Source: CAD feature listing. Evaluate the final solid. Frame: model axes, mm. Face numbers are marked on the shaded views. A direction names the side the tool comes from. Give positions to 0.01 mm unless a question says otherwise; leave off trailing zeros. Order: outer loops, then holes, each group sorted by start corner. A loop starts at its lowest first (then second) coordinate and runs counter-clockwise, first axis right, second up. Notation, with made-up numbers: (37.25, 13) - (78.25, 13) arc R23 ccw to (78.25, 42) - close; hole circle Ø7 at (63, -11.75). An arc over 180 degrees is marked (long way). Answer as CSV lines item,"result".
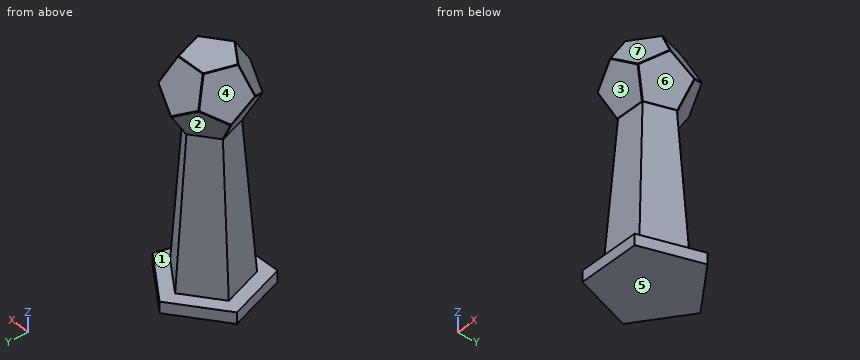
```python
from build123d import *

# Parameters (mm, degrees)
F1_DEPTH      = 2
F1_DEPTH_BACK = 2
F4_ANGLE      = -116.51
F5_COUNT      = 5
F8_ANGLE      = -116.51
F9_COUNT      = 5
F14_ANGLE     = -116.51
F20_DEPTH     = 30


with BuildPart() as f1:
    # F0 (on Top) → F1 (new body, two sides)
    with BuildSketch(Plane.XY) as f1_sk:
        Polygon((38.2616896409, -52.6626978685), (61.9087143061, 20.1153606465), (0, 65.094674444), (-61.9087143061, 20.1153606465), (-38.2616896409, -52.6626978685), align=None)
    extrude(amount=-F1_DEPTH)
    extrude(f1_sk.sketch, amount=F1_DEPTH_BACK)


with BuildPart() as f3_1:
    # F3: copy of F1
    add(f1.part)


with BuildPart() as f3_1_1:
    # F4: moved
    add(f3_1.part.rotate(Axis((30.954357153, 42.6050175452, 0), (0.8090169944, -0.5877852523, 0)), F4_ANGLE))


with BuildPart() as f5_1:
    # F5: instance of F3_1
    add(f3_1_1.part.rotate(Axis((0, 0, 53.0848614872), (0, 0, 1)), 1 * 360 / F5_COUNT))


with BuildPart() as f5_2:
    # F5: instance of F3_1
    add(f3_1_1.part.rotate(Axis((0, 0, 53.0848614872), (0, 0, 1)), 2 * 360 / F5_COUNT))


with BuildPart() as f5_3:
    # F5: instance of F3_1
    add(f3_1_1.part.rotate(Axis((0, 0, 53.0848614872), (0, 0, 1)), 3 * 360 / F5_COUNT))


with BuildPart() as f5_4:
    # F5: instance of F3_1
    add(f3_1_1.part.rotate(Axis((0, 0, 53.0848614872), (0, 0, 1)), 4 * 360 / F5_COUNT))


with BuildPart() as f7_1:
    # F7: copy of F3_1
    add(f3_1_1.part)


with BuildPart() as f7_1_1:
    # F8: moved
    add(f7_1.part.rotate(Axis((80.9914244955, 58.8124345203, 85.250931688), (0.5002969823, -0.6877821992, -0.525983437)), F8_ANGLE))


with BuildPart() as f9_1:
    # F9: instance of F7_1
    add(f7_1_1.part.rotate(Axis((0, 0, 53.0848614872), (0, 0, 1)), 1 * 360 / F9_COUNT))


with BuildPart() as f9_2:
    # F9: instance of F7_1
    add(f7_1_1.part.rotate(Axis((0, 0, 53.0848614872), (0, 0, 1)), 2 * 360 / F9_COUNT))


with BuildPart() as f9_3:
    # F9: instance of F7_1
    add(f7_1_1.part.rotate(Axis((0, 0, 53.0848614872), (0, 0, 1)), 3 * 360 / F9_COUNT))


with BuildPart() as f9_4:
    # F9: instance of F7_1
    add(f7_1_1.part.rotate(Axis((0, 0, 53.0848614872), (0, 0, 1)), 4 * 360 / F9_COUNT))


with BuildPart() as f11_1:
    # F11: copy of F9_4
    add(f9_4.part)


with BuildPart() as f12_1:
    # F12: copy of F7_1
    add(f7_1_1.part)


with BuildPart() as f12_1_1:
    # F14: moved
    add(f12_1.part.rotate(Axis((49.7991616985, 16.4611398873, 170.3695933153), (0.3085369287, -0.9512120135, -0.0008179145)), F14_ANGLE))


with BuildPart() as f1_1:
    add(f1.part)

    # F15 (on face) → F18 section 0
    with BuildSketch(Plane(origin=(0, 0, -2), x_dir=(1, 0, 0), z_dir=(0, 0, -1))):
        Polygon((61.9087143061, -20.1153606465), (38.2616896409, 52.6626978685), (-38.2616896409, 52.6626978685), (-61.9087143061, -20.1153606465), (0, -65.094674444), align=None)
    # F17 (on offset) → F18 section 1
    with BuildSketch(Plane.XY.offset(-400)):
        Polygon((-56.358693348, -77.5710865855), (56.358693348, -77.5710865855), (91.1902813985, 29.6295185314), (0, 95.8831361082), (-91.1902813985, 29.6295185314), align=None)
    loft()

    add(f3_1_1.part)  # F20 merges F3_1

    add(f5_1.part)  # F20 merges F5_1

    add(f5_2.part)  # F20 merges F5_2

    add(f5_3.part)  # F20 merges F5_3

    add(f5_4.part)  # F20 merges F5_4

    add(f7_1_1.part)  # F20 merges F7_1

    add(f9_1.part)  # F20 merges F9_1

    add(f9_2.part)  # F20 merges F9_2

    add(f9_3.part)  # F20 merges F9_3

    add(f9_4.part)  # F20 merges F9_4

    add(f12_1_1.part)  # F20 merges F12_1
    # F19 (on offset) → F20 (join)
    with BuildSketch(Plane.XY.offset(-400)):
        Polygon((-81.073921122, -111.5886792541), (81.073921122, -111.5886792541), (131.1803599767, 42.6230827153), (0, 137.9311930774), (-131.1803599767, 42.6230827153), align=None)
    extrude(amount=-F20_DEPTH)


solid = f1_1.part
```
(1) Contact query for flat-ended pins moving along their axis: pin 1 (12 mm diameter, centred on y = 51, z = -333.5, fed in from -X); pin 2 (10 mm diameter, centred on y = 28.5, z = 58.5, fed in from +X); pin 3 (6 mm diameter, centred on y = -16, z = 31, fed in from -X). Output: stop coordinate, or through.
Completed:
pin 1,"x = -62.98"
pin 2,"x = 100.75"
pin 3,"x = -70.63"
(2) Cut plane A-A (z = 126). Return loops of the section in (x, y).
Completed:
outline,"(-90.13, -28.19) - (-88.07, -28.54) - (-89.52, -30.02) - (-1.04, -94.43) - (-0.07, -92.58) - (0.89, -94.41) - (89.49, -30.17) - (88.03, -28.68) - (90.07, -28.33) - (56.35, 75.78) - (54.48, 74.86) - (54.77, 76.91) - (-54.66, 77.01) - (-54.36, 74.94) - (-56.22, 75.86) - close; hole (-85.23, -27.61) - (-0.08, -89.59) - (85.18, -27.76) - (52.73, 72.43) - (-52.59, 72.53) - close"
(3) Access query for the marked faces 1, 2, 3 and 4. Directions: +Z, -Z, +X, -X, +Y, -Y. A direction counts if a zero-diameter tool reaches every point of the face in a straight line with its end or side. Return the directions, or none.
Completed:
face 1,"none"
face 2,"-X, +Y"
face 3,"+X, -X, -Y"
face 4,"+Z, -X, +Y"
(4) Cut plane B-B (z = 34). Return loops of the section in (x, y), then the cut area to 3 significant figures.
Completed:
outline,"(-84.08, 26.23) - (-52.6, -70.64) - (-50.61, -69.66) - (-50.93, -71.86) - (50.93, -71.86) - (50.61, -69.66) - (52.6, -70.64) - (84.08, 26.23) - (81.89, 26.61) - (83.44, 28.2) - (1.03, 88.07) - (0, 86.11) - (-1.03, 88.07) - (-83.44, 28.2) - (-81.89, 26.61) - close; hole (-79.22, 25.74) - (-48.96, -67.39) - (48.96, -67.39) - (79.22, 25.74) - (0, 83.29) - close"
area,"2,250 mm²"
(5) Ray query, line 1 (Z direction, x = -87.5, y = -30); line 2 (Z direction, x = -4, y = -39.5); line 3 (Z direction, x = -43, y = -81.5). Return the intervals inside material, ascending. Write a range as from..to.
Completed:
line 1,"-430..-400, 75.36..84.32, 119.49..128.4"
line 2,"-430..2, 168.17..172.17"
line 3,"-430..-400, 53.33..62.29, 88.71..97.63"
(6) Cut plane C-C (x = 110.5). Return loops of the section in (y, z).
Completed:
outline,"(-21.02, -430) - (57.65, -430) - (57.65, -400) - (-21.02, -400) - close"
(7) Mould query, pull axis Z, two halves, no side actions, for the marked faces 5, 6 and 7. Classes: released by +Z, released by -Z, zero draft, split by the parting line, or undercut.
Completed:
face 5,"released by -Z"
face 6,"undercut"
face 7,"released by +Z"
